The model under review builds one solid part; all positions refer to its coordinate system, in mm. A direction names the side the tool comes from. Round coordinates to 2 decimals unless told otherwise and drop trailing zeros. Order: outer loops, then holes, each group sorted by start corner. A loop starts at its lowest first (then second) coordinate and runs counter-clockwise, first axis right, second up. Notation, with made-up numbers: M 89,-1 L 108,-1 A30 ccw 108,32 Z; hole C 67.25,84 d3. An arc over 180 degrees is marked long. Use a Markdown table: item, result. Add a question column.
1. Insertion check: P1, Ø5, axis at x = 11.79, z = 11.02, coming from the +Y side; P2, Ø7.5, axis at x = 5.5, y = 25.5, coming from the -Z side. Each pin has a flat end and moves straight along its axis. Give the tip position at first contact, or say it passes through.
2. Consider section B-B on y = 22. State the section outline as (x, z) points, then the cut area to 3 significant figures.
3. The part is to be moulded in two halves that separate along Y. For faces 4 (the flat face through (7, 6, 15)), 5 (the flat face through (7, 12, 8)), 6 (the cylindrical face through (12.011, 9.465, 9.034)), say which applies: +Y half, -Y half, draft (parallel to the pull), parting line (faces both ways), or undercut.
4. Consider section C-C on x = 7.5. State the section outline as (y, z) points.
5. Consider section D-D on z = 13. State the section outline as (x, y) points.
6. To check wall thickness, follow probe 1 along X at (y, z) = (8.3, 13); probe 2 along Y at (x, z) = (8.75, 4.75); probe 3 along Z at (x, y) = (9.5, 28). State the ranges of each line that lie inside material, in increasing order.
7. Consider section A-A on z = 6.75. State the section outline as (x, y) points.
8. For faces 1 (the flat face through (7, 5, 8)), 2 (the flat face through (5.7, 19.9, 15)), 3 (the cylindrical face through (9, 24, 18)), list the 3-axis set-ups (+Z, -Z, +X, -X, +Y, -Y) from which the entire face can be reached by the end or side of a thin tool; tool diameter is ignored.
from build123d import *

# Parameters (mm, degrees)
ESTRUSIONE_ESTRUSIONE1_DEPTH = 15
SCHIZZO5_W                   = 15
SCHIZZO5_H                   = 20
SCHIZZO5_R                   = 2.5
ESTRUSIONE_ESTRUSIONE2_DEPTH = 5
SCHIZZO6_R                   = 2
TAGLIO_ESTRUSIONE2_DEPTH     = 12
SCHIZZO4_R                   = 1.5
TAGLIO_ESTRUSIONE1_DEPTH     = 12


with BuildPart() as part:
    # Schizzo1 → Estrusione-Estrusione1 (new body)
    with BuildSketch(Plane(origin=(0, 0, 0), x_dir=(0, 0, -1), z_dir=(1, 0, 0))):
        Polygon((0, 0), (-20, 0), (-20, 12), (0, 12), (0, 7), (-15, 7), (-15, 5), (0, 5), align=None)
    extrude(amount=ESTRUSIONE_ESTRUSIONE1_DEPTH)

    # Schizzo5 → Estrusione-Estrusione2 (add)
    with BuildSketch(Plane.XY.offset(20)):
        with Locations((7.5, 22)):
            Rectangle(SCHIZZO5_W, SCHIZZO5_H)
        with Locations((7.5, 22)):
            Circle(SCHIZZO5_R, mode=Mode.SUBTRACT)
    extrude(amount=-ESTRUSIONE_ESTRUSIONE2_DEPTH)

    # Schizzo6 → Taglio-Estrusione2 (cut)
    with BuildSketch(Plane.XZ):
        with Locations((3.21150116, 11.021600653)):
            Circle(SCHIZZO6_R)
        with Locations((11.78849884, 11.021600653)):
            Circle(SCHIZZO6_R)
    extrude(amount=-TAGLIO_ESTRUSIONE2_DEPTH, mode=Mode.SUBTRACT)

    # Schizzo4 → Taglio-Estrusione1 (cut)
    with BuildSketch(Plane.XZ):
        with Locations((3.5, 13)):
            Circle(SCHIZZO4_R)
        with Locations((11.5, 13)):
            Circle(SCHIZZO4_R)
    extrude(amount=-TAGLIO_ESTRUSIONE1_DEPTH, mode=Mode.SUBTRACT)


solid = part.part
Answer block:
| question | item | result |
|---|---|---|
| 1 | P1 | y = 12 |
| 1 | P2 | z = 15 |
| 2 | outline | M 0,15 L 5,15 L 5,20 L 0,20 Z; M 10,15 L 15,15 L 15,20 L 10,20 Z |
| 2 | area | 50.0 mm^2 |
| 3 | face 4 | undercut |
| 3 | face 5 | +Y half |
| 3 | face 6 | draft |
| 4 | outline | M 0,0 L 5,0 L 5,15 L 7,15 L 7,0 L 12,0 L 12,15 L 19.5,15 L 19.5,20 L 0,20 Z; M 24.5,15 L 32,15 L 32,20 L 24.5,20 Z |
| 5 | outline | M 0,0 L 2,0 L 2,5 L 0,5 Z; M 0,7 L 2,7 L 2,12 L 0,12 Z; M 5,0 L 10,0 L 10,5 L 5,5 Z; M 5,7 L 10,7 L 10,12 L 5,12 Z; M 13,0 L 15,0 L 15,5 L 13,5 Z; M 13,7 L 15,7 L 15,12 L 13,12 Z |
| 6 | probe 1 | 0 to 2, 5 to 10, 13 to 15 |
| 6 | probe 2 | 0 to 5, 7 to 12 |
| 6 | probe 3 | 15 to 20 |
| 7 | outline | M 0,0 L 15,0 L 15,5 L 0,5 Z; M 0,7 L 15,7 L 15,12 L 0,12 Z |
| 8 | face 1 | -Z, +X, -X |
| 8 | face 2 | -Z, +X, -X, +Y |
| 8 | face 3 | +Z, -Z |
